```python
from build123d import *

# Parameters (mm, degrees)
SKETCH1_W            = 284.48
SKETCH1_H            = 101.6
BOSS_EXTRUDE1_DEPTH  = 55.88
SKETCH2_W            = 76.042421072
SKETCH2_H            = 101.6
BOSS_EXTRUDE2_DEPTH  = 274.32
SKETCH3_W            = 68.280460578
SKETCH3_H            = 6.35
CUT_EXTRUDE1_DEPTH   = 147.32
SKETCH4_R            = 3.175
CUT_EXTRUDE2_DEPTH   = 274.32
SKETCH5_W            = 25.4
SKETCH5_H            = 50.8
BOSS_EXTRUDE4_DEPTH  = 38.1
SKETCH6_W            = 29.665893143
SKETCH6_H            = 25.4
BOSS_EXTRUDE5_DEPTH  = 50.8
SKETCH7_W            = 76.2
SKETCH7_H            = 62.556650574
BOSS_EXTRUDE6_DEPTH  = 93.98
SKETCH8_R            = 6.35
BOSS_EXTRUDE7_DEPTH  = 7.62
SKETCH9_W            = 50.8
SKETCH9_H            = 50.8
BOSS_EXTRUDE8_DEPTH  = 7.62
SKETCH11_W           = 88.356231919
SKETCH11_H           = 63.5
BOSS_EXTRUDE9_DEPTH  = 44.45
SKETCH13_R           = 6.35
BOSS_EXTRUDE10_DEPTH = 7.62
SKETCH14_W           = 50.8
SKETCH14_H           = 50.8
BOSS_EXTRUDE11_DEPTH = 7.62
SKETCH15_R           = 3.175
BOSS_EXTRUDE12_DEPTH = 19.05
CHAMFER2_SIZE        = 6.35


with BuildPart() as part:
    # Sketch1 → Boss-Extrude1 (new body)
    with BuildSketch(Plane(origin=(0, 0, 0), x_dir=(1, 0, 0), z_dir=(0, 1, 0))):
        with Locations((142.24, 50.8)):
            Rectangle(SKETCH1_W, SKETCH1_H)
    extrude(amount=BOSS_EXTRUDE1_DEPTH)

    # Sketch2 → Boss-Extrude2 (add)
    with BuildSketch(Plane(origin=(0, 55.88, 0), x_dir=(1, 0, 0), z_dir=(0, 1, 0))):
        with Locations((114.337337429, 50.8)):
            Rectangle(SKETCH2_W, SKETCH2_H)
    extrude(amount=BOSS_EXTRUDE2_DEPTH)

    # Sketch3 → Cut-Extrude1 (cut)
    with BuildSketch(Plane(origin=(0, 203.2, 0), x_dir=(1, 0, 0), z_dir=(0, 1, 0))):
        with Locations((92.975896604, 33.655)):
            Rectangle(SKETCH3_W, SKETCH3_H)
        with Locations((92.975896604, 67.945)):
            Rectangle(SKETCH3_W, SKETCH3_H)
    extrude(amount=-CUT_EXTRUDE1_DEPTH, mode=Mode.SUBTRACT)

    # Sketch4 → Cut-Extrude2 (cut)
    with BuildSketch(Plane.ZY.offset(-127.116126893)):
        with Locations((-33.655, 98.425)):
            Circle(SKETCH4_R)
        with Locations((-67.945, 64.135)):
            Circle(SKETCH4_R)
    extrude(amount=-CUT_EXTRUDE2_DEPTH, mode=Mode.SUBTRACT)

    # Sketch5 → Boss-Extrude4 (add)
    with BuildSketch(Plane.ZY.offset(-76.316126893)):
        with Locations((-88.9, 81.28)):
            Rectangle(SKETCH5_W, SKETCH5_H)
        with Locations((-12.7, 81.28)):
            Rectangle(SKETCH5_W, SKETCH5_H)
    extrude(amount=BOSS_EXTRUDE4_DEPTH)

    # Sketch6 → Boss-Extrude5 (add)
    with BuildSketch(Plane(origin=(0, 55.88, 0), x_dir=(1, 0, 0), z_dir=(0, 1, 0))):
        with Locations((14.832946572, 88.9)):
            Rectangle(SKETCH6_W, SKETCH6_H)
        with Locations((14.832946572, 12.7)):
            Rectangle(SKETCH6_W, SKETCH6_H)
    extrude(amount=BOSS_EXTRUDE5_DEPTH)

    # Sketch7 → Boss-Extrude6 (add)
    with BuildSketch(Plane.ZY.offset(-20.32)):
        with Locations((-50.8, 75.401674713)):
            Rectangle(SKETCH7_W, SKETCH7_H)
    extrude(amount=BOSS_EXTRUDE6_DEPTH)

    # Sketch8 → Boss-Extrude7 (add)
    with BuildSketch(Plane(origin=(20.32, 0, 0), x_dir=(0, 0, -1), z_dir=(1, 0, 0))):
        with Locations((50.8, 81.28)):
            Circle(SKETCH8_R)
    extrude(amount=BOSS_EXTRUDE7_DEPTH)

    # Sketch9 → Boss-Extrude8 (add)
    with BuildSketch(Plane(origin=(27.94, 0, 0), x_dir=(0, 0, -1), z_dir=(1, 0, 0))):
        with Locations((50.8, 81.28)):
            Rectangle(SKETCH9_W, SKETCH9_H)
    extrude(amount=BOSS_EXTRUDE8_DEPTH)

    # Sketch11 → Boss-Extrude9 (add)
    with BuildSketch(Plane(origin=(0, 55.88, 0), x_dir=(1, 0, 0), z_dir=(0, 1, 0))):
        with Locations((240.30188404, 50.8)):
            Rectangle(SKETCH11_W, SKETCH11_H)
    extrude(amount=BOSS_EXTRUDE9_DEPTH)

    # Sketch13 → Boss-Extrude10 (add)
    with BuildSketch(Plane.ZY.offset(-196.123768081)):
        with Locations((-50.8, 78.105)):
            Circle(SKETCH13_R)
    extrude(amount=BOSS_EXTRUDE10_DEPTH)

    # Sketch14 → Boss-Extrude11 (add)
    with BuildSketch(Plane.ZY.offset(-188.503768081)):
        with Locations((-50.8, 81.28)):
            Rectangle(SKETCH14_W, SKETCH14_H)
    extrude(amount=BOSS_EXTRUDE11_DEPTH)

    # Sketch15 → Boss-Extrude12 (add)
    with BuildSketch(Plane.ZY.offset(-180.883768081)):
        with Locations((-33.655, 98.425)):
            Circle(SKETCH15_R)
        with Locations((-67.945, 64.135)):
            Circle(SKETCH15_R)
    extrude(amount=BOSS_EXTRUDE12_DEPTH)

    # Chamfer2
    chamfer2_edges = [part.edges().sort_by_distance(p)[0] for p in [
        (-36.83, 44.123349426, -88.9),
        (-36.83, 106.68, -88.9),
        (-36.83, 106.68, -12.7),
        (-36.83, 44.123349426, -12.7),
        (240.301884041, 100.33, -82.55),
        (240.301884041, 100.33, -19.05),
    ]]
    chamfer(chamfer2_edges, length=CHAMFER2_SIZE)


solid = part.part
```
Input: part model. Units: mm. Frame: model coordinates. A direction names the side the tool comes from. Round coordinates to 2 decimals unless told otherwise and drop trailing zeros. Order: outer loops, then holes, each group sorted by start corner. A loop starts at its lowest first (then second) coordinate and runs counter-clockwise, first axis right, second up. Notation, with made-up numbers: (-25.5, 12) - (-21.5, 12) arc R29 cw to (-21.5, 42) - close; hole circle Ø6 at (50, 53.5). An arc over 180 degrees is marked (long way). One line per question, with ' | ' between items. Start each with the question number.
1) Cut plane D-D, the plane x = -26.5. Return the cut outline in (y, z), then the cut area to 3 significant figures.
2) Ray query, probe 1 along Z at (x, y) = (104.5, 113.5); probe 2 along X at (y, z) = (96.5, -87.5); probe 3 along Z at (x, y) = (43, 92.5). Return the intervals inside material, ascending.
3) Cut plane B-B, the plane z = -50.8. Give the number of separate pieces and of enclosed holes in the cut face, then the cut area to 3 significant figures.
4) Cut plane C-C, the plane y = 127.5. Return the cut outline in (x, z), then the cut area to 3 significant figures.
5) Set-up query: faces 1 (the flat face through (185, 106.68, -51)), 2 (the cylindrical face through (24.077, 75.646, -53.73)), 3 (the flat face through (58, 81, -76.2)), 4 (the flat face through (38.216, 82, -89)). Return all of +Z, -Z, +X, -X, +Y, -Y with unobstructed straight access to the full face (end or side cutting, diameter ignored); none if empty.
6) Pull-direction query (Z, two-part tool) for faces 5 (the flat face through (58, 106.68, -89)), 6 (the flat face through (58, 81, -25.4)), 7 (the flat face through (109, 126, -101.6)); classes: +Z half, -Z half, draft (parallel to the pull), parting line (faces both ways), or undercut.
7) Contact query for flat-ended pins moving along their axis: P1, Ø2.5, axis at x = 185, y = 88, coming from the -Z side; P2, Ø10, axis at y = 250, z = -39.5, coming from the -X side; P3, Ø5, axis at y = 277, z = -47.5, coming from the +X side. Output: stop coordinate, or through.
8) Cut plane A-A, the plane x = 170. Return the cut outline in (y, z) (3 decimals).
Worked out:
1) outline: (44.12, -82.55) - (50.47, -88.9) - (100.33, -88.9) - (106.68, -82.55) - (106.68, -19.05) - (100.33, -12.7) - (50.47, -12.7) - (44.12, -19.05) - close | area: 4,690 mm^2
2) probe 1: z = -101.6 to -71.12, -64.77 to -36.83, -30.48 to 0 | probe 2: x = -73.66 to 29.67, 38.22 to 152.36 | probe 3: z = -101.6 to -76.2, -25.4 to 0
3) separate pieces: 1 | enclosed holes: 2 | area: 47,300 mm^2
4) outline: (76.32, -101.6) - (152.36, -101.6) - (152.36, 0) - (76.32, 0) - (76.32, -30.48) - (127.12, -30.48) - (127.12, -36.83) - (76.32, -36.83) - (76.32, -64.77) - (127.12, -64.77) - (127.12, -71.12) - (76.32, -71.12) - close | area: 7,080 mm^2
5) face 1: +Z, -Z, +X, +Y | face 2: none | face 3: +Y | face 4: +Z, -Z, +Y
6) face 5: draft | face 6: undercut | face 7: -Z half
7) P1: stops at z = -76.2 | P2: stops at x = 76.32 | P3: stops at x = 152.36
8) outline: (0, -101.6) - (55.88, -101.6) - (55.88, 0) - (0, 0) - close; circle Ø6.35 at (64.135, -67.945); circle Ø6.35 at (98.425, -33.655)
